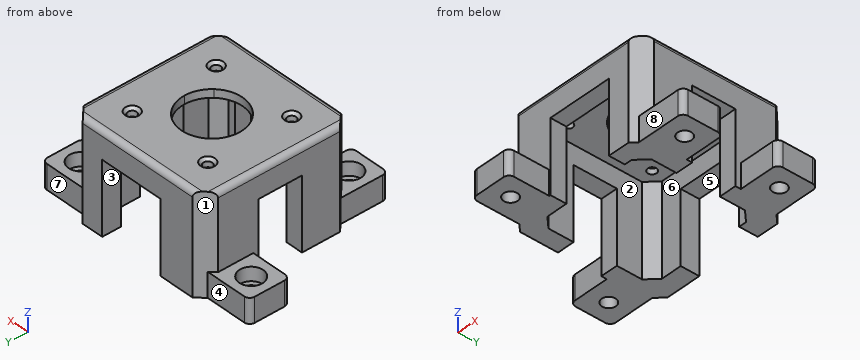
from build123d import *

# Parameters (mm, degrees)
SKETCH2_W           = 55
SKETCH2_H           = 55
BOSS_EXTRUDE1_DEPTH = 33.6
BOSS_EXTRUDE2_DEPTH = 3
SKETCH4_W           = 15
SKETCH4_H           = 15
SKETCH4_R           = 2.6
BOSS_EXTRUDE3_DEPTH = 9
CUT_EXTRUDE1_START  = -5
SKETCH6_R           = 4.4
SKETCH6_R_2         = 2.6
CUT_EXTRUDE1_DEPTH  = 5
CHAMFER1_SIZE       = 5
FILLET4_R           = 2
SKETCH7_W           = 24
SKETCH7_H           = 26.6
CUT_EXTRUDE2_DEPTH  = 67
SKETCH8_W           = 26.6
SKETCH8_H           = 16
CUT_EXTRUDE3_DEPTH  = 67
SKETCH10_R          = 1.65
CUT_EXTRUDE4_DEPTH  = 10
CHAMFER2_SIZE       = 1


with BuildPart() as part:
    # Sketch2 → Boss-Extrude1 (new body)
    with BuildSketch(Plane.XY):
        with Locations((0, 0.476186899)):
            Rectangle(SKETCH2_W, SKETCH2_H)
        Polygon((21.118377871, -17.280631787), (21.118377871, 17.280631787), (17.280631787, 21.118377871), (-17.280631787, 21.118377871), (-21.118377871, 17.280631787), (-21.118377871, -17.280631787), (-17.280631787, -21.118377871), (17.280631787, -21.118377871), align=None, mode=Mode.SUBTRACT)
    extrude(amount=BOSS_EXTRUDE1_DEPTH)

    # Sketch3 → Boss-Extrude2 (add)
    with BuildSketch(Plane.XY.offset(33.6)):
        with BuildLine():
            Line((-7.954951288, 8.431138187), (-18.961411379, 19.437598278))
            Line((-18.961411379, 19.437598278), (-21.118377871, 17.280631787))
            Line((-21.118377871, 17.280631787), (-21.118377871, -17.280631787))
            Line((-21.118377871, -17.280631787), (-19.437598278, -18.961411379))
            Line((-19.437598278, -18.961411379), (-7.954951288, -7.478764389))
            ThreePointArc((-7.954951288, -7.478764389), (-11.25, 0.476186899), (-7.954951288, 8.431138187))
        make_face()
        with BuildLine():
            Line((-7.954951288, -7.478764389), (-19.437598278, -18.961411379))
            Line((-19.437598278, -18.961411379), (-17.280631787, -21.118377871))
            Line((-17.280631787, -21.118377871), (17.280631787, -21.118377871))
            Line((17.280631787, -21.118377871), (19.437598278, -18.961411379))
            Line((19.437598278, -18.961411379), (7.954951288, -7.478764389))
            ThreePointArc((7.954951288, -7.478764389), (0, -10.773813101), (-7.954951288, -7.478764389))
        make_face()
        with BuildLine():
            Line((21.118377871, 17.280631787), (18.961411379, 19.437598278))
            Line((18.961411379, 19.437598278), (7.954951288, 8.431138187))
            ThreePointArc((7.954951288, 8.431138187), (10.393644741, 4.781375513), (11.25, 0.476186899))
            ThreePointArc((11.25, 0.476186899), (10.393644741, -3.829001715), (7.954951288, -7.478764389))
            Line((7.954951288, -7.478764389), (19.437598278, -18.961411379))
            Line((19.437598278, -18.961411379), (21.118377871, -17.280631787))
            Line((21.118377871, -17.280631787), (21.118377871, 17.280631787))
        make_face()
        with BuildLine():
            Line((-17.280631787, 21.118377871), (-18.961411379, 19.437598278))
            Line((-18.961411379, 19.437598278), (-7.954951288, 8.431138187))
            ThreePointArc((-7.954951288, 8.431138187), (0, 11.726186899), (7.954951288, 8.431138187))
            Line((7.954951288, 8.431138187), (18.961411379, 19.437598278))
            Line((18.961411379, 19.437598278), (17.280631787, 21.118377871))
            Line((17.280631787, 21.118377871), (-17.280631787, 21.118377871))
        make_face()
        Polygon((-18.961411379, 19.437598278), (-27.5, 27.976186899), (-27.5, -27.023813101), (-19.437598278, -18.961411379), (-21.118377871, -17.280631787), (-21.118377871, 17.280631787), align=None)
        Polygon((-19.437598278, -18.961411379), (-27.5, -27.023813101), (27.5, -27.023813101), (19.437598278, -18.961411379), (17.280631787, -21.118377871), (-17.280631787, -21.118377871), align=None)
        Polygon((27.5, -27.023813101), (27.5, 27.976186899), (18.961411379, 19.437598278), (21.118377871, 17.280631787), (21.118377871, -17.280631787), (19.437598278, -18.961411379), align=None)
        Polygon((27.5, 27.976186899), (-27.5, 27.976186899), (-18.961411379, 19.437598278), (-17.280631787, 21.118377871), (17.280631787, 21.118377871), (18.961411379, 19.437598278), align=None)
    extrude(amount=BOSS_EXTRUDE2_DEPTH)

    # Sketch4 → Boss-Extrude3 (add)
    # profile 1 of 4: a face of its own
    with BuildSketch(Plane(origin=(0, 0, 0), x_dir=(-1, 0, 0), z_dir=(0, 0, -1))):
        with Locations((-35, 17.5)):
            Rectangle(SKETCH4_W, SKETCH4_H)
        with Locations((-35, 17.5)):
            Circle(SKETCH4_R, mode=Mode.SUBTRACT)
    # profile 2 of 4: a face of its own
    with BuildSketch(Plane(origin=(0, 0, 0), x_dir=(-1, 0, 0), z_dir=(0, 0, -1))):
        with Locations((35, 17.5)):
            Rectangle(SKETCH4_W, SKETCH4_H)
        with Locations((35, 17.5)):
            Circle(SKETCH4_R, mode=Mode.SUBTRACT)
    # profile 3 of 4: a face of its own
    with BuildSketch(Plane(origin=(0, 0, 0), x_dir=(-1, 0, 0), z_dir=(0, 0, -1))):
        with Locations((-35, -17.5)):
            Rectangle(SKETCH4_W, SKETCH4_H)
        with Locations((-35, -17.5)):
            Circle(SKETCH4_R, mode=Mode.SUBTRACT)
    # profile 4 of 4: a face of its own
    with BuildSketch(Plane(origin=(0, 0, 0), x_dir=(-1, 0, 0), z_dir=(0, 0, -1))):
        with Locations((17.5, -34.523813101)):
            Rectangle(SKETCH4_W, SKETCH4_H)
        with Locations((17.5, -34.523813101)):
            Circle(SKETCH4_R, mode=Mode.SUBTRACT)
    extrude(amount=-BOSS_EXTRUDE3_DEPTH)

    # Sketch6 → Cut-Extrude1 (cut)
    # profile 1 of 4: a face of its own
    with BuildSketch(Plane.XY.offset(9).offset(CUT_EXTRUDE1_START)):
        with Locations((-17.5, -34.523813101)):
            Circle(SKETCH6_R)
    # profile 2 of 4: a face of its own
    with BuildSketch(Plane.XY.offset(9).offset(CUT_EXTRUDE1_START)):
        with Locations((-35, 17.5)):
            Circle(SKETCH6_R)
    # profile 3 of 4: a face of its own
    with BuildSketch(Plane.XY.offset(9).offset(CUT_EXTRUDE1_START)):
        with Locations((35, -17.5)):
            Circle(SKETCH6_R)
        with Locations(Location((35, -17.5, 0), (0, 0, 180))):
            Circle(SKETCH6_R_2, mode=Mode.SUBTRACT)
    # profile 4 of 4: a face of its own
    with BuildSketch(Plane.XY.offset(9).offset(CUT_EXTRUDE1_START)):
        with Locations((35, 17.5)):
            Circle(SKETCH6_R)
    extrude(amount=CUT_EXTRUDE1_DEPTH, mode=Mode.SUBTRACT)

    # Chamfer1
    chamfer1_edges = [part.edges().sort_by_distance(p)[0] for p in [
        (27.5, -27.023813101, 18.3),
        (-27.5, -27.023813101, 18.3),
        (27.5, 27.976186899, 18.3),
        (-27.5, 27.976186899, 18.3),
    ]]
    chamfer(chamfer1_edges, length=CHAMFER1_SIZE)

    # Fillet4
    fillet4_edges = [part.edges().sort_by_distance(p)[0] for p in [
        (0, 27.976186899, 36.6),
        (27.5, 0.476186899, 36.6),
        (0, -27.023813101, 36.6),
        (-27.5, 0.476186899, 36.6),
        (-25, -42.023813101, 4.5),
        (-10, -42.023813101, 4.5),
        (-42.5, 10, 4.5),
        (-42.5, 25, 4.5),
        (42.5, -25, 4.5),
        (42.5, -10, 4.5),
        (42.5, 10, 4.5),
        (42.5, 25, 4.5),
    ]]
    fillet(fillet4_edges, radius=FILLET4_R)

    # Sketch7 → Cut-Extrude2 (cut)
    with BuildSketch(Plane.XZ.offset(27.023813101)):
        with Locations((2.5, 13.3)):
            Rectangle(SKETCH7_W, SKETCH7_H)
    extrude(amount=-CUT_EXTRUDE2_DEPTH, mode=Mode.SUBTRACT)

    # Sketch8 → Cut-Extrude3 (cut)
    with BuildSketch(Plane.ZY.offset(27.5)):
        with Locations((13.3, 0)):
            Rectangle(SKETCH8_W, SKETCH8_H)
    extrude(amount=-CUT_EXTRUDE3_DEPTH, mode=Mode.SUBTRACT)


with BuildPart() as body_2:
    # Mirror2: mirrored copy
    add(part.part.mirror(Plane(origin=(-25, -42.023813101, 9), x_dir=(0, 0, 1), z_dir=(0, 1, 0))))


with BuildPart() as body_2_2:
    # Mirror3: mirrored copy
    add(body_2.part.mirror(Plane(origin=(-1.737426519, -112.023813101, 20.07988243), x_dir=(0, 0, 1), z_dir=(0, -1, 0))))

    # Sketch10 → Cut-Extrude4 (cut)
    with BuildSketch(Plane.XY.offset(36.6)):
        with Locations((-15.5, -124.023813101)):
            Circle(SKETCH10_R)
        with Locations((15.5, -124.023813101)):
            Circle(SKETCH10_R)
        with Locations((15.5, -155.023813101)):
            Circle(SKETCH10_R)
        with Locations((-15.5, -155.023813101)):
            Circle(SKETCH10_R)
    extrude(amount=-CUT_EXTRUDE4_DEPTH, mode=Mode.SUBTRACT)

    # Chamfer2
    chamfer2_edges = [body_2_2.edges().sort_by_distance(p)[0] for p in [
        (-17.15, -155.023813101, 36.6),
        (13.85, -155.023813101, 36.6),
        (13.85, -124.023813101, 36.6),
        (-17.15, -124.023813101, 36.6),
    ]]
    chamfer(chamfer2_edges, length=CHAMFER2_SIZE)


solid = body_2_2.part
Can you work these out from the model? Positions are in its coordinate system, mm. Face numbers are marked on the shaded views. A direction names the side the tool comes from. Give positions to 0.01 mm unless a question says otherwise; leave off trailing zeros. Order: outer loops, then holes, each group sorted by start corner. A loop starts at its lowest first (then second) coordinate and runs counter-clockwise, first axis right, second up. Notation, with made-up numbers: (-9, -35.75) - (25, -35.75) arc R34 cw to (25, -4.75) - close; hole circle Ø10 at (36.25, 59.25). An arc over 180 degrees is marked (long way). Write each question's results on one line, items separated by ' | '.
1) Suppose I cut it at C-C, the plane z = 28. Write out the boundary of the cut face in (x, y), then the cut area to 3 significant figures.
Final values:
outline: (-27.5, -162.02) - (-22.5, -167.02) - (22.5, -167.02) - (27.5, -162.02) - (27.5, -117.02) - (22.5, -112.02) - (-22.5, -112.02) - (-27.5, -117.02) - close; hole (-21.12, -157.28) - (-17.28, -161.12) - (17.28, -161.12) - (21.12, -157.28) - (21.12, -122.72) - (17.28, -118.88) - (-17.28, -118.88) - (-21.12, -122.72) - close | area: 1,220 mm^2
2) Suppose I cut it at D-D, the plane x = -35. Write out the boundary of the cut face in (y, z).
Final values:
outline: (-130, 0) - (-125.1, 0) - (-125.1, 4) - (-126.9, 4) - (-126.9, 9) - (-130, 9) - close; (-119.9, 0) - (-115, 0) - (-115, 9) - (-118.1, 9) - (-118.1, 4) - (-119.9, 4) - close
3) I'm going to push flat-ended pins straight in: pin 1 Ø1 at (x, z) = (-27, 13) entering from +Y; pin 2 Ø4.5 at (x, z) = (-35.5, 6) entering from +Y; pin 3 Ø10.5 at (y, z) = (-147, 9.5) entering from -X. Where does each tip first touch, or does it pass through?
Final values:
pin 1: stops at y = -116.02 | pin 2: stops at y = -115 | pin 3: stops at x = -27.5
4) If we mould it in two halves opening along Y, with no side actions, what happens to the marked faces 1, 2 and 3? For each: pulls with the +Y half, pulls with the -Y half, needs draft (parallel to the pull), parting line crosses it, or undercut.
Final values:
face 1: pulls with the +Y half | face 2: undercut | face 3: needs draft
5) Suppose I cut it at B-B, the plane z = 15.5. Give the number of separate pieces and of enclosed holes in the cut face, then the cut area to 3 significant figures.
Final values:
separate pieces: 4 | enclosed holes: 0 | area: 710 mm^2
6) Suppose I cut it at A-A, the plane x = 15.5. Write out the boundary of the cut face in (y, z).
Final values:
outline: (-167.02, 0) - (-161.12, 0) - (-161.12, 33.6) - (-156.67, 33.6) - (-156.67, 35.6) - (-157.67, 36.6) - (-165.02, 36.6) arc R2 ccw to (-167.02, 34.6) - close; (-153.37, 33.6) - (-125.67, 33.6) - (-125.67, 35.6) - (-126.67, 36.6) - (-152.37, 36.6) - (-153.37, 35.6) - close; (-122.37, 33.6) - (-118.88, 33.6) - (-118.88, 0) - (-112.02, 0) - (-112.02, 34.6) arc R2 ccw to (-114.02, 36.6) - (-121.37, 36.6) - (-122.37, 35.6) - close
7) On a 3-axis mill with a long thin cutter (end or side, diameter ignored), from which of +Z, -Z, +X, -X, +Y, -Y can I reach the whole of each face in a straight line? I mean the marked faces 4, 5, 6, 7 and 8. Say none if no direction works.
Final values:
face 4: +Z, -Z, -X, +Y | face 5: -Z, +Y, -Y | face 6: -Z | face 7: +Z, -Z, +X, +Y | face 8: +Z, -Z, +X, -Y
8) Please list where these lines run through material, in increasing order: line 1 along Y through (x, z) = (35, 5.15); line 2 along Y through (x, z) = (35, 2.55); line 3 along Y through (x, z) = (-4.5, 28). Write a range as [from, to].
Final values:
line 1: y = [-165, -161.9], [-153.1, -150], [-130, -126.9], [-118.1, -115] | line 2: y = [-165, -160.1], [-154.9, -150], [-130, -125.1], [-119.9, -115] | line 3: y = [-167.02, -161.12], [-118.88, -112.02]
